Could you check a few things on this model? Use its own coordinates, in mm. A direction names the side the tool comes from. Round coordinates to 2 decimals unless told otherwise and drop trailing zeros. Order: outer loops, then holes, each group sorted by start corner. A loop starts at its lowest first (then second) coordinate and runs counter-clockwise, first axis right, second up. Notation, with made-up numbers: M -3,0.5 L 55,0.5 A15 ccw 55,26.5 Z; hole C -5,77.25 d1. An arc over 180 degrees is marked long. Write each question's results on one line, items separated by ' | '. Start each with the question number.
1. Suppose I cut it at B-B on y = -22. Write out the boundary of the cut face in (x, z), and give its area (3 significant figures).
2. Suppose I cut it at D-D on z = 0.95. Write out the boundary of the cut face in (x, y).
3. Suppose I cut it at C-C on x = 6. Write out the boundary of the cut face in (y, z).
4. I'm going to push flat-ended pins straight in: pin 1 (15 mm diameter, centred on x = 2, y = 7, fed in from +Z); pin 2 (3 mm diameter, centred on x = -13, y = -17, fed in from +Z); pin 3 (0.7 mm diameter, centred on x = 5.5, z = 1, fed in from +Y). Where does each tip first touch, or does it pass through?
5. Suppose I cut it at A-A on x = 0. Write out the boundary of the cut face in (y, z).
6. Please list where these lines run through material, in increasing order: L1, parallel to X at y = 5, z = 0.2; L2, parallel to Y at x = -2, z = 1.25; L3, parallel to Z at x = -11, y = 13.5.
7. For faces 4 (the cylindrical face through (0.1, -10, 0.2)), 5 (the cylindrical face through (-12.235, -14.678, 0.197)), 6 (the flat face through (-7, -1, 0.4)), 7 (the cylindrical face through (12.38, -14.47, 0.2)), which set-ups out of +Z, -Z, +X, -X, +Y, -Y let a thin tool reach every point of the face, with its end or its side?
8. We'd pull the mould along X, two halves only. Please class faces 1 (the flat face through (16.5, -34, 1)), 2 (the flat face through (0, -33, 0)), 3 (the cylindrical face through (-0.1, 10, 0.2)): released by +X, released by -X, zero draft, split by the parting line, or undercut.
from build123d import *

# Parameters (mm, degrees)
BOSS_EXTRUDE1_DEPTH = 0.4
SKETCH2_W           = 33
SKETCH2_H           = 19
BOSS_EXTRUDE2_DEPTH = 1.4
BOSS_EXTRUDE3_START = -0.001
SKETCH3_W           = 0.4
SKETCH3_H           = 6
BOSS_EXTRUDE3_DEPTH = 0.401


with BuildPart() as part:
    # Sketch1 → Boss-Extrude1 (new body)
    with BuildSketch(Plane.XY):
        with BuildLine():
            Line((15, 6), (15, -6))
            ThreePointArc((15, -6), (0, -21), (-15, -6))
            Line((-15, -6), (-15, 6))
            ThreePointArc((-15, 6), (0, 21), (15, 6))
        make_face()
        with BuildLine():
            Line((5, 5), (5, -5))
            ThreePointArc((5, -5), (0, -10), (-5, -5))
            Line((-5, -5), (-5, 5))
            ThreePointArc((-5, 5), (0, 10), (5, 5))
        make_face(mode=Mode.SUBTRACT)
    extrude(amount=BOSS_EXTRUDE1_DEPTH)



with BuildPart() as body_2:
    # Sketch2 → Boss-Extrude2 (new body)
    with BuildSketch(Plane.XY):
        with Locations((0, -33.5)):
            Rectangle(SKETCH2_W, SKETCH2_H)
    extrude(amount=BOSS_EXTRUDE2_DEPTH)


with BuildPart() as part_1:
    add(part.part)

    add(body_2.part)  # Boss-Extrude3 merges body 2
    # Sketch3 → Boss-Extrude3 (add)
    with BuildSketch(Plane.XY.offset(BOSS_EXTRUDE3_START)):
        with Locations((5, -21.260407867)):
            Rectangle(SKETCH3_W, SKETCH3_H)
        with Locations((-5, -21.22123599)):
            Rectangle(SKETCH3_W, SKETCH3_H)
    extrude(amount=BOSS_EXTRUDE3_DEPTH)


solid = part_1.part
Filled sheet:
1) outline: M -5.2,0 L -4.8,0 L -4.8,0.4 L -5.2,0.4 Z; M 4.8,0 L 5.2,0 L 5.2,0.4 L 4.8,0.4 Z | area: 0.321 mm^2
2) outline: M -16.5,-43 L 16.5,-43 L 16.5,-24 L -16.5,-24 Z
3) outline: M -43,0 L -24,0 L -24,1.4 L -43,1.4 Z; M -19.75,0 L 19.75,0 L 19.75,0.4 L -19.75,0.4 Z
4) pin 1: stops at z = 0.4 | pin 2: passes through | pin 3: stops at y = -24
5) outline: M -43,0 L -24,0 L -24,1.4 L -43,1.4 Z; M -21,0 L -10,0 L -10,0.4 L -21,0.4 Z; M 10,0 L 21,0 L 21,0.4 L 10,0.4 Z
6) L1: x = -15 to -5, 5 to 15 | L2: y = -43 to -24 | L3: z = 0 to 0.4
7) face 4: +Z, -Z | face 5: +Z, -Z, -X | face 6: +Z, +X, -X, +Y | face 7: +Z, -Z, +X
8) face 1: released by +X | face 2: zero draft | face 3: undercut
